For this review, use the dimensioned drawing (mm, ordinates from the lowest corner) and the shaded views. A direction names the side the tool comes from. Give positions to 0.01 mm unless a question says otherwise; leave off trailing zeros. Write each loop counter-clockwise with the first axis right and the second up, starting at its lowest first coordinate (ties: lowest second). Pieces come first, ordered by that corner, then holes. Notation, with made-up numbers: (-30, 76) - (-3, 76) arc R11 cw to (-3, 82) - close; hole circle Ø10 at (25.5, 17). An arc over 180 degrees is marked (long way). Use a Markdown table: item, result. Add a question column.
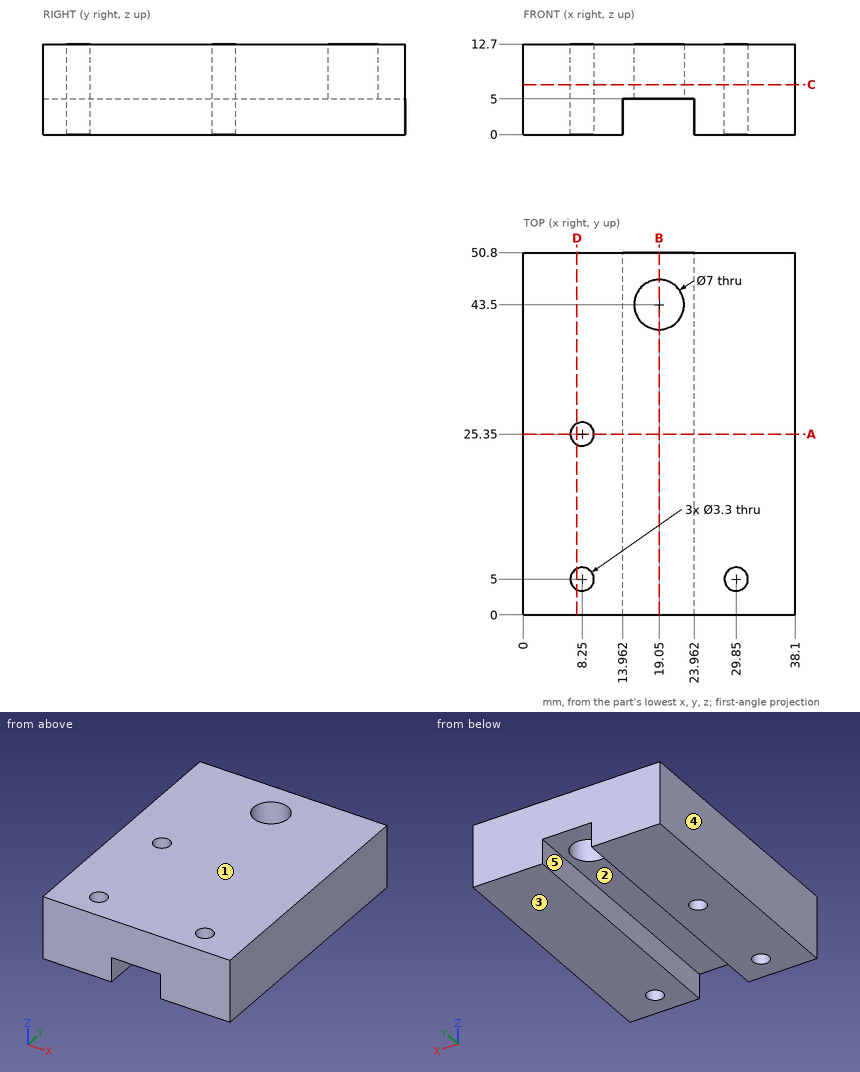
(1) Add section A-A (y = 25.35). State the section outline as (x, z) points.
(2) Add section D-D (x = 7.5). State the section outline as (y, z) points.
(3) For line 1 along Y through (x, z) = (8.25, 4.25); line 2 along X through (y, z) = (25.5, 11); line 3 along X through (y, z) = (24.5, 3) (1 decimal), list the stretches that pass through material, from the lowest coordinate up.
(4) Add section C-C (z = 7). State the section outline as (x, y) points.
(5) Add section B-B (x = 19.05). State the section outline as (y, z) points, and give its area (3 significant figures).
(6) Mouldability with a two-part tool opening along X and no side actions: class the marked faces 3, 4 and 5 as +X half, -X half, draft (parallel to the pull), parting line (faces both ways), or undercut.
(7) Tool access review of the marked faces 1 and 2: name each direction out of +Z, -Z, +X, -X, +Y, -Y from which nothing blocks a thin tool from reaching the whole face with its end or side.
Answers follow:
| question | item | result |
|---|---|---|
| 1 | outline | (0, 0) - (6.6, 0) - (6.6, 12.7) - (0, 12.7) - close; (9.9, 0) - (13.96, 0) - (13.96, 5) - (23.96, 5) - (23.96, 0) - (38.1, 0) - (38.1, 12.7) - (9.9, 12.7) - close |
| 2 | outline | (0, 0) - (3.53, 0) - (3.53, 12.7) - (0, 12.7) - close; (6.47, 0) - (23.88, 0) - (23.88, 12.7) - (6.47, 12.7) - close; (26.82, 0) - (50.8, 0) - (50.8, 12.7) - (26.82, 12.7) - close |
| 3 | line 1 | 0 to 3.35, 6.65 to 23.7, 27 to 50.8 |
| 3 | line 2 | 0 to 6.61, 9.89 to 38.1 |
| 3 | line 3 | 0 to 6.8, 9.7 to 14, 24 to 38.1 |
| 4 | outline | (0, 0) - (38.1, 0) - (38.1, 50.8) - (0, 50.8) - close; hole circle Ø3.3 at (8.25, 5); hole circle Ø3.3 at (8.25, 25.35); hole circle Ø7 at (19.05, 43.5); hole circle Ø3.3 at (29.85, 5) |
| 5 | outline | (0, 5) - (40, 5) - (40, 12.7) - (0, 12.7) - close; (47, 5) - (50.8, 5) - (50.8, 12.7) - (47, 12.7) - close |
| 5 | area | 337 mm^2 |
| 6 | face 3 | draft |
| 6 | face 4 | -X half |
| 6 | face 5 | undercut |
| 7 | face 1 | +Z, +X, -X, +Y, -Y |
| 7 | face 2 | -Z, +Y, -Y |
